from build123d import *

# Parameters (mm, degrees)
F0_R     = 1.45
F0_R_2   = 5
F0_W     = 6
F0_H     = 8
F1_DEPTH = 6
F2_DEPTH = 1.5
F0_R_3   = 2.75
F3_DEPTH = 5


with BuildPart() as f1:
    # F0 (on Top) → F1 (new body)
    with BuildSketch(Plane.XY):
        Polygon((3, -10), (10, -10), (10, 10), (-10, 10), (-10, -10), (-3, -10), (-3, -2), (3, -2), align=None)
        with Locations((6.4, -6)):
            Circle(F0_R, mode=Mode.SUBTRACT)
        with Locations((0, 4)):
            Circle(F0_R_2, mode=Mode.SUBTRACT)
        with Locations((0, -6)):
            Rectangle(F0_W, F0_H)
    extrude(amount=F1_DEPTH)

    # F0 (on Top) → F2 (join)
    with BuildSketch(Plane.XY):
        with Locations((0, -6)):
            Rectangle(F0_W, F0_H)
    extrude(amount=-F2_DEPTH)

    # F0 (on Top) → F3 (join)
    with BuildSketch(Plane.XY):
        with Locations((0, 4)):
            Circle(F0_R_2)
        with Locations((0, 4)):
            Circle(F0_R_3, mode=Mode.SUBTRACT)
    extrude(amount=F3_DEPTH)


solid = f1.part
Input: part model. Units: mm. Frame: model coordinates. A direction names the side the tool comes from. Give positions to 0.01 mm unless a question says otherwise; leave off trailing zeros. Loops run counter-clockwise (first coordinate to the right, second up) from the corner with the lowest first, then second, coordinate; pieces in that order, holes last. Notation, with made-up numbers: M 19,73 L 48,73 A26 cw 48,90 Z; hole C -1.75,63.5 d9. An arc over 180 degrees is marked long. Use one line per item in the form item = value.
1. Reachability of faces 4 (the face through (2.2, 1.8, 5)), 5 (the face through (0, -2, -1)), 6 (the face through (3, -6, -1)) from +Z, -Z, +X, -X, +Y, -Y: full face, straight path, thin tool, end or side. Return the list, or none.
Numbers:
face_4 = +Z
face_5 = -Z, +X, -X, +Y
face_6 = -Z, +X, +Y, -Y
2. Section query A-A, the plane x = 6.4. Return the cut outline in (y, z), and give its area (3 significant figures).
Numbers:
outline = M -10,0 L -7.45,0 L -7.45,6 L -10,6 Z; M -4.55,0 L 10,0 L 10,6 L -4.55,6 Z
area = 103 mm²
3. Section query B-B, the plane y = 4. Return the cut outline in (x, z), and give its area (3 significant figures).
Numbers:
outline = M -10,0 L -2.75,0 L -2.75,5 L -5,5 L -5,6 L -10,6 Z; M 2.75,0 L 10,0 L 10,6 L 5,6 L 5,5 L 2.75,5 Z
area = 82.5 mm²
4. Section query D-D, the plane x = 0. Return the cut outline in (y, z).
Numbers:
outline = M -10,-1.5 L -2,-1.5 L -2,0 L 1.25,0 L 1.25,5 L -1,5 L -1,6 L -10,6 Z; M 6.75,0 L 10,0 L 10,6 L 9,6 L 9,5 L 6.75,5 Z
5. Pull-direction query (Y, two-part tool) for faces 1 (the face through (-0.596, 1.315, 2.465)), 2 (the face through (0, -10, 3)), 3 (the face through (-3, -6, -1)); classes: released by +Y, released by -Y, zero draft, split by the parting line, or undercut.
Numbers:
face_1 = undercut
face_2 = released by -Y
face_3 = zero draft
6. First-contact query: pin 1 (7 mm diameter, centred on x = 0, y = 4, fed in from -Z); pin 2 (0.8 mm diameter, centred on y = -6, z = -1, fed in from +X); pin 3 (1.6 mm diameter, centred on y = -4.5, z = -1, fed in from -X). Flat tips, straight axial feed; report the tip coordinate or a pass-through.
Numbers:
pin_1 = 0
pin_2 = 3
pin_3 = -3
7. Line query: L1, parallel to Y at x = 0, z = 2.95; L2, parallel to Y at x = 0, z = 5.75; L3, parallel to Z at x = -7.25, y = -6.5. Output: solid intervals per line, ascending.
Numbers:
L1 = -10 to 1.25, 6.75 to 10
L2 = -10 to -1, 9 to 10
L3 = 0 to 6
8. Section query C-C, the plane z = 3.5. Return the cut outline in (x, y), and give its area (3 significant figures).
Numbers:
outline = M -10,-10 L 10,-10 L 10,10 L -10,10 Z; hole C 0,4 d5.5; hole C 6.4,-6 d2.9
area = 370 mm²
